Could you check a few things on this model? Use its own coordinates, in mm. A direction names the side the tool comes from. Round coordinates to 2 decimals unless told otherwise and drop trailing zeros. Loops run counter-clockwise (first coordinate to the right, second up) from the corner with the lowest first, then second, coordinate; pieces in that order, holes last. Notation, with made-up numbers: (-22, 3) -> (36, 3) arc R24 cw to (36, 39) -> close; hole circle Ø6 at (-27, -0.5). An arc over 180 degrees is marked (long way). Write each question's results on one line, items separated by ' | '.
from build123d import *

# Parameters (mm, degrees)
SKETCH1_W                            = 104
SKETCH1_H                            = 58
SKETCH1_W_2                          = 11.5
SKETCH1_H_2                          = 7.75
MODULAR_MAIN_BODY_DEPTH              = 17.75
FRONT_CUT_OUT_DEPTH                  = 107.43853951
SKETCH5_R                            = 3.5
MODULAR_INTERFACE_DEEP_CUT_OUT_DEPTH = 10
FILLET1_R                            = 1
FILLET3_R                            = 1


with BuildPart() as part:
    # Sketch1 → modular_main_body (new body)
    with BuildSketch(Plane.XY):
        with Locations((-35.464851186, 13.154761905)):
            Rectangle(SKETCH1_W, SKETCH1_H)
        with Locations((-53.214851186, 30.279761905)):
            Rectangle(SKETCH1_W_2, SKETCH1_H_2, mode=Mode.SUBTRACT)
    extrude(amount=MODULAR_MAIN_BODY_DEPTH)

    # Sketch2 → front_cut_out (cut, through all)
    with BuildSketch(Plane.XZ.offset(15.845238095)):
        with BuildLine():
            Line((-23.964851186, 17.75), (-13.964851186, 14.8))
            Line((-13.964851186, 14.8), (10.035148814, 14.8))
            ThreePointArc((10.035148814, 14.8), (15.960148814, 8.875), (10.035148814, 2.95))
            Line((10.035148814, 2.95), (-13.964851186, 2.95))
            Line((-13.964851186, 2.95), (-23.964851186, 0))
            Line((-23.964851186, 0), (16.535148814, 0))
            Line((16.535148814, 0), (16.535148814, 17.75))
            Line((16.535148814, 17.75), (-23.964851186, 17.75))
        make_face()
    extrude(amount=-FRONT_CUT_OUT_DEPTH, mode=Mode.SUBTRACT)

    # Sketch5 → modular_interface_deep_cut_out (cut)
    with BuildSketch(Plane(origin=(0, 42.154761905, 0), x_dir=(1, 0, 0), z_dir=(0, 1, 0))):
        with Locations(Location((-78.464851186, -8.875, 0), (0, 0, 180))):
            Circle(SKETCH5_R)
        with Locations(Location((-27.464851186, -8.875, 0), (0, 0, 180))):
            Circle(SKETCH5_R)
        with Locations(Location((-10.464851186, -8.875, 0), (0, 0, 180))):
            Circle(SKETCH5_R)
        with Locations(Location((6.535148814, -8.875, 0), (0, 0, 180))):
            Circle(SKETCH5_R)
    extrude(amount=-MODULAR_INTERFACE_DEEP_CUT_OUT_DEPTH, mode=Mode.SUBTRACT)

    # Fillet1
    fillet1_edges = [part.edges().sort_by_distance(p)[0] for p in [
        (-18.964851186, -15.845238095, 16.275),
        (-1.964851186, -15.845238095, 14.8),
        (15.960148814, -15.845238095, 8.875),
        (-1.964851186, -15.845238095, 2.95),
        (-18.964851186, -15.845238095, 1.475),
        (-55.714851186, -15.845238095, 0),
        (-55.714851186, -15.845238095, 17.75),
        (-87.464851186, -15.845238095, 8.875),
    ]]
    fillet(fillet1_edges, radius=FILLET1_R)

    # Fillet3
    # the kernel refuses this fillet: 1 mm, written as the material it takes off along each edge
    with BuildSketch(Plane(origin=(-86.464851186, -14.845238095, 16.75), x_dir=(0, 0, 1), z_dir=(-1, 0, 0))) as fillet3_piece_1_section:
        Polygon((0, 0), (FILLET3_R, 0), (FILLET3_R, -FILLET3_R), (0, -FILLET3_R), align=None)
    fillet3_piece_1 = extrude(amount=FILLET3_R, mode=Mode.PRIVATE)
    fillet3_piece_1 = fillet3_piece_1 - Plane(origin=(-86.464851186, -14.845238095, 16.75), x_dir=(0, 0.7071067811865475, -0.7071067811865475), z_dir=(-1, 0, 0)) * Sphere(FILLET3_R, mode=Mode.PRIVATE)
    add(fillet3_piece_1, mode=Mode.SUBTRACT)
    with BuildSketch(Plane(origin=(-86.464851186, -14.845238095, 1), x_dir=(-1, 0, 0), z_dir=(0, 0, -1))) as fillet3_piece_2_section:
        Polygon((0, 0), (FILLET3_R, 0), (FILLET3_R, -FILLET3_R), (0, -FILLET3_R), align=None)
    fillet3_piece_2 = extrude(amount=FILLET3_R, mode=Mode.PRIVATE)
    fillet3_piece_2 = fillet3_piece_2 - Plane(origin=(-86.464851186, -14.845238095, 1), x_dir=(0.7071067811865475, 0.7071067811865475, 0), z_dir=(0, 0, -1)) * Sphere(FILLET3_R, mode=Mode.PRIVATE)
    add(fillet3_piece_2, mode=Mode.SUBTRACT)
    with BuildSketch(Plane(origin=(-87.464851186, -14.845238095, 17.75), x_dir=(0, 0, -1), z_dir=(0, 1, 0)), Plane(origin=(-87.464851186, -14.845238095, 0), x_dir=(1, 0, 0), z_dir=(0, 1, 0))) as fillet3_piece_3:
        with BuildLine():
            CenterArc((FILLET3_R, -FILLET3_R), FILLET3_R, 90, 90)
            Line((0, -FILLET3_R), (0, 0))
            Line((0, 0), (FILLET3_R, 0))
        make_face()
    extrude(amount=59.5, mode=Mode.SUBTRACT)


solid = part.part
1) I'm going to push flat-ended pins straight in: pin 1 (7 mm diameter, centred on x = 3.5, y = 5.5, fed in from +Z); pin 2 (2 mm diameter, centred on x = 6, z = 9, fed in from +Y); pin 3 (5 mm diameter, centred on y = 22.5, z = 16, fed in from +X). Where does each tip first touch, or does it pass through?
Model answer:
pin 1: stops at z = 14.8 | pin 2: stops at y = 32.15 | pin 3: stops at x = 13.74
2) If we mould it in two halves opening along Z, with no side actions, what happens to faces 5 (the cylindrical face through (-30.698, 37.225, 7.534)), 6 (the flat face through (-19.035, 13.256, 16.296)), 7 (the flat face through (-48, 42.155, 9)), 8 (the cylindrical face through (-7.687, 37.225, 6.745))? For each: released by +Z, released by -Z, zero draft, split by the parting line, or undercut.
Model answer:
face 5: undercut | face 6: released by +Z | face 7: zero draft | face 8: undercut
3) I want a section at D-D, the plane x = -76.5. Write out the boundary of the cut face in (y, z), plus the area to 3 significant figures.
Model answer:
outline: (-15.85, 1) arc R1 ccw to (-14.85, 0) -> (42.15, 0) -> (42.15, 5.98) -> (32.15, 5.98) -> (32.15, 11.77) -> (42.15, 11.77) -> (42.15, 17.75) -> (-14.85, 17.75) arc R1 ccw to (-15.85, 16.75) -> close | area: 971 mm2
4) I need wall thicknesses on line 1 (Y direction, x = -52, z = 9.25); line 2 (Z direction, x = -3, y = 14); line 3 (Y direction, x = 9, z = 6.5). Which ranges of each line are inside material? Lowest first, please.
Model answer:
line 1: y = -15.85 to 26.4, 34.15 to 42.15 | line 2: z = 2.95 to 14.8 | line 3: y = -15.85 to 32.15
5) I want a section at B-B, the plane y = -9. Write out the boundary of the cut face in (x, z) (3 decimals).
Model answer:
outline: (-87.465, 1) arc R1 ccw to (-86.465, 0) -> (-23.965, 0) -> (-13.965, 2.95) -> (10.035, 2.95) arc R5.925 ccw to (10.035, 14.8) -> (-13.965, 14.8) -> (-23.965, 17.75) -> (-86.465, 17.75) arc R1 ccw to (-87.465, 16.75) -> close
6) I want a section at A-A, the plane x = -52.5. Write out the boundary of the cut face in (y, z).
Model answer:
outline: (-15.85, 1) arc R1 ccw to (-14.85, 0) -> (26.4, 0) -> (26.4, 17.75) -> (-14.85, 17.75) arc R1 ccw to (-15.85, 16.75) -> close; (34.15, 0) -> (42.15, 0) -> (42.15, 17.75) -> (34.15, 17.75) -> close
7) For faces 1 (the flat face through (7, 32.155, 9)), 2 (the flat face through (-2, 13, 2.95)), 3 (the flat face through (-47.465, 30, 9)), 4 (the flat face through (-2, 13, 14.8)), which set-ups out of +Z, -Z, +X, -X, +Y, -Y let a thin tool reach every point of the face, with its end or its side?
Model answer:
face 1: +Y | face 2: -Z, +X, +Y, -Y | face 3: +Z, -Z | face 4: +Z, +X, +Y, -Y
8) I want a section at C-C, the plane y = 36. Write out the boundary of the cut face in (x, z) (3 decimals), plus the area to 3 significant figures.
Model answer:
outline: (-87.465, 1) arc R1 ccw to (-86.465, 0) -> (-23.965, 0) -> (-13.965, 2.95) -> (10.035, 2.95) arc R5.925 ccw to (10.035, 14.8) -> (-13.965, 14.8) -> (-23.965, 17.75) -> (-86.465, 17.75) arc R1 ccw to (-87.465, 16.75) -> close; hole circle Ø7 at (-78.465, 8.875); hole circle Ø7 at (-27.465, 8.875); hole circle Ø7 at (-10.465, 8.875); hole circle Ø7 at (6.535, 8.875) | area: 1,460 mm2
